```python
from build123d import *

# Parameters (mm, degrees)
ESQUISSE1_W                       = 35
ESQUISSE1_H                       = 35
BOSS_EXTRU_1_DEPTH                = 34.8
ESQUISSE2_R                       = 11
BOSS_EXTRU_2_DEPTH                = 2
ESQUISSE3_R                       = 2.5
BOSS_EXTRU_3_DEPTH                = 22
ESQUISSE8_W                       = 1.389274908
ESQUISSE8_H                       = 3
ENL_V_MAT_EXTRU_2_DEPTH           = 16.6
DIAM_TRE_DU_PER_AGE_3_0_3_1_D     = 3
DIAM_TRE_DU_PER_AGE_3_0_3_1_DEPTH = 4.2
DIAM_TRE_DU_PER_AGE_3_0_3_1_TIP   = 0.901290929
CONG_1_R                          = 2.5
ENL_V_MAT_EXTRU_1_DEPTH           = 7.5
ESQUISSE5_R                       = 0.7
ESQUISSE5_R_2                     = 0.654723083
BOSS_EXTRU_4_DEPTH                = 10


with BuildPart() as part:
    # Esquisse1 → Boss.-Extru.1 (new body)
    with BuildSketch(Plane(origin=(0, 0, 0), x_dir=(1, 0, 0), z_dir=(0, 1, 0))):
        Rectangle(ESQUISSE1_W, ESQUISSE1_H)
    extrude(amount=BOSS_EXTRU_1_DEPTH)

    # Esquisse2 → Boss.-Extru.2 (add)
    with BuildSketch(Plane(origin=(0, 34.8, 0), x_dir=(1, 0, 0), z_dir=(0, 1, 0))):
        with Locations(Location((0, 0, 0), (0, 0, 270))):
            Circle(ESQUISSE2_R)
    extrude(amount=BOSS_EXTRU_2_DEPTH)

    # Esquisse3 → Boss.-Extru.3 (add)
    with BuildSketch(Plane(origin=(0, 36.8, 0), x_dir=(1, 0, 0), z_dir=(0, 1, 0))):
        with Locations(Location((0, 0, 0), (0, 0, 270))):
            Circle(ESQUISSE3_R)
    extrude(amount=BOSS_EXTRU_3_DEPTH)

    # Esquisse8 → Enlèv. mat.-Extru.2 (cut)
    with BuildSketch(Plane(origin=(0, 58.8, 0), x_dir=(1, 0, 0), z_dir=(0, 1, 0))):
        with Locations((-2.694637454, 0)):
            Rectangle(ESQUISSE8_W, ESQUISSE8_H)
    extrude(amount=-ENL_V_MAT_EXTRU_2_DEPTH, mode=Mode.SUBTRACT)

    # Diamètre du perçage Ø3.0 (3)1
    with Locations(Plane(origin=(0, 34.8, 0), x_dir=(1, 0, 0), z_dir=(0, 1, 0))):
        with Locations((-13, 13), (13, 13), (13, -13), (-13, -13)):
            Hole(DIAM_TRE_DU_PER_AGE_3_0_3_1_D / 2, depth=DIAM_TRE_DU_PER_AGE_3_0_3_1_DEPTH)
            with Locations((0, 0, -(DIAM_TRE_DU_PER_AGE_3_0_3_1_DEPTH + DIAM_TRE_DU_PER_AGE_3_0_3_1_TIP / 2))):  # 118° drill point
                Cone(0, DIAM_TRE_DU_PER_AGE_3_0_3_1_D / 2, DIAM_TRE_DU_PER_AGE_3_0_3_1_TIP, mode=Mode.SUBTRACT)

    # Congé1
    cong_1_edges = [part.edges().sort_by_distance(p)[0] for p in [
        (-17.5, 17.4, -17.5),
        (17.5, 17.4, -17.5),
        (17.5, 17.4, 17.5),
        (-17.5, 17.4, 17.5),
    ]]
    fillet(cong_1_edges, radius=CONG_1_R)

    # Esquisse4 → Enlèv. mat.-Extru.1 (cut, symmetric)
    with BuildSketch(Plane(origin=(0, 17.4, 0), x_dir=(1, 0, 0), z_dir=(0, 1, 0))):
        Polygon((-12.5, 17.5), (-17.5, 12.5), (-17.5, 17.5), align=None)
        Polygon((17.5, 17.5), (12.5, 17.5), (17.5, 12.5), align=None)
        Polygon((12.5, -17.5), (17.5, -12.5), (17.5, -17.5), align=None)
        Polygon((-17.5, -17.5), (-12.5, -17.5), (-17.5, -12.5), align=None)
    extrude(amount=ENL_V_MAT_EXTRU_1_DEPTH, both=True, mode=Mode.SUBTRACT)

    # Esquisse5 → Boss.-Extru.4 (add)
    with BuildSketch(Plane.ZY.offset(17.5)):
        with Locations(Location((-1, 7, 0), (0, 0, 180))):
            Circle(ESQUISSE5_R)
        with Locations(Location((-1, 5, 0), (0, 0, 180))):
            Circle(ESQUISSE5_R_2)
        with Locations(Location((1, 5, 0), (0, 0, 180))):
            Circle(ESQUISSE5_R_2)
        with Locations(Location((1, 7, 0), (0, 0, 180))):
            Circle(ESQUISSE5_R)
    extrude(amount=BOSS_EXTRU_4_DEPTH)


solid = part.part
```
Can you work these out from the model? Positions are in its coordinate system, mm. A direction names the side the tool comes from. Round coordinates to 2 decimals unless told otherwise and drop trailing zeros. Loops run counter-clockwise (first coordinate to the right, second up) from the corner with the lowest first, then second, coordinate; pieces in that order, holes last. Notation, with made-up numbers: (-35.75, 50.25) -> (18.25, 50.25) arc R20 cw to (18.25, 88.25) -> close; hole circle Ø4 at (-23.5, -4.5). An arc over 180 degrees is marked (long way). Answer in a Markdown table with one row per item.
Item 1: Suppose I cut it at B-B, the plane x = 0. List the corners of the cut face in (y, z) for me, plus the area to 3 significant figures.
Answer block:
| item | result |
|---|---|
| outline | (0, -17.5) -> (34.8, -17.5) -> (34.8, -11) -> (36.8, -11) -> (36.8, -2.5) -> (58.8, -2.5) -> (58.8, 2.5) -> (36.8, 2.5) -> (36.8, 11) -> (34.8, 11) -> (34.8, 17.5) -> (0, 17.5) -> close |
| area | 1,370 mm² |
Item 2: Will these pins go through, and if not, where does the flat tip stop? P1, Ø1, axis at x = -17.5, z = 8, coming from the +Y side; P2, Ø2.5, axis at x = 13, z = 13, coming from the +Y side; P3, Ø1.5, axis at y = 47.5, z = -0.5, coming from the -X side.
Answer block:
| item | result |
|---|---|
| P1 | y = 34.8 |
| P2 | y = 30.45 |
| P3 | x = -2 |
Item 3: On a 3-axis mill with a long thin cutter (end or side, diameter ignored), from which of +Z, -Z, +X, -X, +Y, -Y can I reach the whole of each face in a straight line? I mean faces 4 (the flat face through (-16, 9.9, -16)), 5 (the cylindrical face through (-22.43, 5.58, -1.3)), 6 (the cylindrical face through (14.5, 32.67, 12.93)), 7 (the flat face through (-15, 18, 15)), 8 (the flat face through (15, 17, 15)). Say none if no direction works.
Answer block:
| item | result |
|---|---|
| face 4 | -Z, -X |
| face 5 | -X |
| face 6 | +Y |
| face 7 | +Z, -X |
| face 8 | +Z, +X |
Item 4: If I drill on probe 1 along X at (y, z) = (32.7, -13); probe 2 along Y at (x, z) = (4, 3.5), over which ranges is the centre line in solid material (lowest first)?
Answer block:
| item | result |
|---|---|
| probe 1 | -17.5 to -14.5, -11.5 to 11.5, 14.5 to 17.5 |
| probe 2 | 0 to 36.8 |
Item 5: Suppose I cut it at A-A, the plane y = 34. List the corners of the cut face in (x, z) for me, plus the area to 3 significant figures.
Answer block:
| item | result |
|---|---|
| outline | (-17.5, -15) arc R2.5 ccw to (-15, -17.5) -> (15, -17.5) arc R2.5 ccw to (17.5, -15) -> (17.5, 15) arc R2.5 ccw to (15, 17.5) -> (-15, 17.5) arc R2.5 ccw to (-17.5, 15) -> close; hole circle Ø3 at (-13, -13); hole circle Ø3 at (-13, 13); hole circle Ø3 at (13, -13); hole circle Ø3 at (13, 13) |
| area | 1,190 mm² |
Item 6: Suppose I cut it at C-C, the plane y = 7. List the corners of the cut face in (x, z) for me, plus the area to 3 significant figures.
Answer block:
| item | result |
|---|---|
| outline | (-27.5, -1.7) -> (-17.5, -1.7) -> (-17.5, -15) arc R2.5 ccw to (-15, -17.5) -> (15, -17.5) arc R2.5 ccw to (17.5, -15) -> (17.5, 15) arc R2.5 ccw to (15, 17.5) -> (-15, 17.5) arc R2.5 ccw to (-17.5, 15) -> (-17.5, 1.7) -> (-27.5, 1.7) -> (-27.5, 0.3) -> (-17.5, 0.3) -> (-17.5, -0.3) -> (-27.5, -0.3) -> close |
| area | 1,250 mm² |
Item 7: We'd pull the mould along Z, two halves only. Please class faces 1 (the flat face through (-16, 9.9, 16)), 2 (the cylindrical face through (16.748, 5.019, 16.787)), 3 (the conical face through (-13.26, 29.855, -13.011)): released by +Z, released by -Z, zero draft, split by the parting line, or undercut.
Answer block:
| item | result |
|---|---|
| face 1 | zero draft |
| face 2 | released by +Z |
| face 3 | undercut |
Item 8: Suppose I cut it at D-D, the plane z = -4.5. List the corners of the cut face in (x, y) for me.
Answer block:
| item | result |
|---|---|
| outline | (-17.5, 0) -> (17.5, 0) -> (17.5, 34.8) -> (10.04, 34.8) -> (10.04, 36.8) -> (-10.04, 36.8) -> (-10.04, 34.8) -> (-17.5, 34.8) -> close |
